Can you work these out from the model? Positions are in its coordinate system, mm. A direction names the side the tool comes from. Coordinates: 2 decimals unless noted, no trailing zeros. Order: outer loops, then holes, each group sorted by start corner. A loop starts at its lowest first (then second) coordinate and runs counter-clockwise, first axis right, second up. Notation, with made-up numbers: (6.25, 80.5) -> (34.25, 80.5) arc R15 cw to (34.25, 104.5) -> close; hole circle Ø10 at (65, -35.5). An arc over 180 degrees is marked (long way). Return JSON: item names as keys, results as strings. Group by question number.
1) Thinking about a two-plate mould opening in Y: for faces 5 (the flat face through (-8.65, 0, 6)), 6 (the cylindrical face through (-9.04, -9, 2.03)), 7 (the flat face through (0, 9.9, 2)), 8 (the flat face through (-9.9, 0, 2)), which applies, +Y half, -Y half, draft (parallel to the pull), parting line (faces both ways), or undercut?
2) If we section it at B-B, the plane y = -4.25: Please give me the cut outline in (x, z), then the cut area to 3 significant figures.
3) If we section it at A-A, the plane x = 0.75: Please give me the cut outline in (y, z).
4) For faces 1 (the flat face through (-8.4, 7, 1)), 2 (the flat face through (4.1, 0, 3)), 3 (the flat face through (8.35, 7, 6)), 4 (the flat face through (0, 9.55, 6)), which set-ups out of +Z, -Z, +X, -X, +Y, -Y let a thin tool reach every point of the face, with its end or its side?
5) If we section it at D-D, the plane z = 3.5: Please give me the cut outline in (x, y).
6) If I drill on probe 1 along Y at (x, z) = (-5.5, 2.5); probe 2 along X at (y, z) = (1, 0.5); probe 3 along Y at (x, z) = (-0.75, 5.5), over which ranges is the centre line in solid material (lowest first)? Write a range as from..to.
7) If we section it at C-C, the plane z = 5.5: Please give me the cut outline in (x, y).
8) For pin 1 (1 mm diameter, centred on y = 7, z = 1, fed in from +X); pin 2 (4 mm diameter, centred on y = 3, z = 1, fed in from -X); pin 3 (1.5 mm diameter, centred on x = -4.5, y = -4, fed in from +Z); pin 4 (0.6 mm diameter, centred on x = -4, z = 6, fed in from +Y), each with a flat end and sliding along its axis, tell me the tip position at first contact or that it passes through.
Autodesk Fusion 360 part; units mm, degrees
sketch "Sketch1" plane through (0, 0, 0) normal (0, 0, 1) x (1, 0, 0)
  line L0 (9.9, 9.9) -> (-9.9, 9.9)
  line L1 (-9.9, 9.9) -> (-9.9, -9.9)
  line L2 (-9.9, -9.9) -> (9.9, -9.9)
  line L3 (9.9, -9.9) -> (9.9, 9.9)
  line L4 (9.9, 9.9) -> (-9.9, -9.9) construction
  line L5 (-9.9, 9.9) -> (9.9, -9.9) construction
  line L6 (11, -11) -> (-11, -11)
  line L7 (-11, -11) -> (-11, 11)
  line L8 (-11, 11) -> (11, 11)
  line L9 (11, 11) -> (11, -11)
  line L10 (11, -11) -> (-11, 11) construction
  line L11 (-11, -11) -> (11, 11) construction
  line L12 (8.9, -8.9) -> (-8.9, -8.9)
  line L13 (-8.9, -8.9) -> (-8.9, 8.9)
  line L14 (-8.9, 8.9) -> (8.9, 8.9)
  line L15 (8.9, 8.9) -> (8.9, -8.9)
  line L16 (8.9, -8.9) -> (-8.9, 8.9) construction
  line L17 (-8.9, -8.9) -> (8.9, 8.9) construction
  line L18 (8.4, -6) -> (-8.4, -6)
  line L19 (-8.4, -6) -> (-8.4, 6)
  line L20 (-8.4, 6) -> (8.4, 6)
  line L21 (8.4, 6) -> (8.4, -6)
  line L22 (8.4, -6) -> (-8.4, 6) construction
  line L23 (-8.4, -6) -> (8.4, 6) construction
  line L24 (8.0957, 8.0957) -> (-8.0957, 8.0957)
  line L25 (-8.0957, 8.0957) -> (-8.0957, -8.0957)
  line L26 (-8.0957, -8.0957) -> (8.0957, -8.0957)
  line L27 (8.0957, -8.0957) -> (8.0957, 8.0957)
  line L28 (8.0957, 8.0957) -> (-8.0957, -8.0957) construction
  line L29 (-8.0957, 8.0957) -> (8.0957, -8.0957) construction
  line L30 (8.9, -0.5) -> (-8.9, -0.5)
  line L31 (-8.9, -0.5) -> (-8.9, 0.5)
  line L32 (-8.9, 0.5) -> (8.9, 0.5)
  line L33 (8.9, 0.5) -> (8.9, -0.5)
  line L34 (8.9, -0.5) -> (-8.9, 0.5) construction
  line L35 (-8.9, -0.5) -> (8.9, 0.5) construction
  dimension "d1" = 19.8
  dimension "d2" = 19.8
  dimension "d3" = 22
  dimension "d4" = 22
  dimension "d5" = 17.8
  dimension "d6" = 17.8
  dimension "d7" = 16.8
  dimension "d8" = 12
  dimension "d53" = 1
extrude "Extrude1" add sketch "Sketch1" along normal blind 1 contours L12 L13 L15 L18 L19 L21 L25 L26 L27 L30 | L15 L21 L30 L32 L33 | L13 L19 L30 L31 L32 | L13 L14 L15 L19 L20 L21 L24 L25 L27 L32 | L18 L25 L26 L27 | L20 L24 L25 L27
extrude "Extrude2" add sketch "Sketch1" along normal blind 4 contours L0 L1 L2 L3
extrude "Extrude3" add sketch "Sketch1" along normal blind 5 contours L6 L7 L8 L9
extrude "Extrude4" cut sketch "Sketch1" along normal blind 4 contours L6 L7 L8 L9
extrude "Extrude5" add 1 faces at (-9.5667, -2.9667, 4) along direction (0, 0, 1) blind 1
fillet "Fillet1" radius 3 1 edges at (9.9, -9.9, 2)
fillet "Fillet2" radius 3 1 edges at (-9.9, -9.9, 2)
fillet "Fillet3" radius 3 2 edges at (-9.9, 9.9, 2) (9.9, 9.9, 2)
fillet "Fillet4" radius 1 4 edges at (-11, -11, 4.5) (-11, 11, 4.5) (11, -11, 4.5) (11, 11, 4.5)
extrude "Extrude6" add 1 faces at (-2.8, -7.9333, 1) along direction (0, 0, 1) blind 5
extrude "Extrude7" cut sketch "Sketch1" along normal blind 3 contours L18 L25 L26 L27 | L20 L24 L25 L27
extrude "Extrude8" cut 1 faces at (-8.0957, 7.3972, 1) along direction (-1, 0, 0) blind 0.304
extrude "Extrude9" cut 1 faces at (8.0957, 6.6986, 1) along direction (1, 0, 0) blind 0.304
extrude "Extrude10" cut 1 faces at (8.0957, -7.3972, 1) along direction (1, 0, 0) blind 0.304
extrude "Extrude11" cut 1 faces at (-8.0957, -6.6986, 1) along direction (-1, 0, 0) blind 0.304
sketch "Sketch2" plane through (8.4, 0, 0) normal (-1, 0, 0) x (0, -1, 0)
  line L0 (-6, 0) -> (6, 0)
  line L1 (6, 0) -> (6, 6)
  line L2 (6, 6) -> (-6, 6)
  line L3 (-6, 6) -> (-6, 0)
  line L4 (-6, 6) -> (6, 6)
  line L5 (6, 6) -> (6, 4.0166)
  line L6 (6, 4.0166) -> (-6, 4.0166)
  line L7 (-6, 4.0166) -> (-6, 6)
extrude "Extrude12" add sketch "Sketch2" along normal blind 1 contours L1 L2 L3 L4 L5 L6 L7
sketch "Sketch3" plane through (-8.4, 0, 0) normal (1, 0, 0) x (0, 1, 0)
  line L0 (-6, 0) -> (6, 0)
  line L1 (6, 0) -> (6, 6)
  line L2 (6, 6) -> (-6, 6)
  line L3 (-6, 6) -> (-6, 0)
  line L4 (-6, 6) -> (6, 6)
  line L5 (6, 6) -> (6, 3.9624)
  line L6 (6, 3.9624) -> (-6, 3.9624)
  line L7 (-6, 3.9624) -> (-6, 6)
extrude "Extrude13" add sketch "Sketch3" along normal blind 1 contours L1 L2 L3 L4 L5 L6 L7
extrude "Extrude14" cut 1 faces at (-2.4667, 7.9333, 6) along direction (0, 0, -1) blind 2
extrude "Extrude15" add 1 faces at (-2.4667, 7.9333, 4) along direction (0, 0, 1) blind 1
sketch "TOP BUTTON GUIDE" plane through (0, 0, 5) normal (0, 0, 1) x (-1, 0, 0)
  line L0 (-8.4, 6) -> (7.4, 6)
  line L1 (7.4, 6) -> (7.4, -6)
  line L2 (7.4, -6) -> (-8.4, -6)
  line L3 (-8.4, -6) -> (-8.4, 6)
  arc A0 (-11, -10) -> (-10, -11) centre (-10, -10) ccw
  line L4 (-10, -11) -> (10, -11)
  arc A1 (10, -11) -> (11, -10) centre (10, -10) ccw
  line L5 (11, -10) -> (11, 10)
  arc A2 (11, 10) -> (10, 11) centre (10, 10) ccw
  line L6 (10, 11) -> (-10, 11)
  arc A3 (-10, 11) -> (-11, 10) centre (-10, 10) ccw
  line L7 (-11, 10) -> (-11, -10)
  line L8 (-8.35, 8.25) -> (8.35, 8.25)
  line L9 (8.35, 8.25) -> (8.35, -8.25)
  line L10 (8.35, -8.25) -> (-8.35, -8.25)
  line L11 (-8.35, -8.25) -> (-8.35, 8.25)
  line L12 (-8.35, 8.25) -> (8.35, -8.25) construction
  line L13 (8.35, 8.25) -> (-8.35, -8.25) construction
  line L14 (-9.15, 9.05) -> (9.15, 9.05)
  line L15 (9.15, 9.05) -> (9.15, -9.05)
  line L16 (9.15, -9.05) -> (-9.15, -9.05)
  line L17 (-9.15, -9.05) -> (-9.15, 9.05)
  line L18 (-9.15, 9.05) -> (9.15, -9.05) construction
  line L19 (9.15, 9.05) -> (-9.15, -9.05) construction
  dimension "d47" = 16.7
  dimension "d48" = 16.5
  dimension "d49" = 18.3
  dimension "d50" = 18.1
extrude "Extrude16" add sketch "TOP BUTTON GUIDE" along normal blind 2 contours L14 L15 L16 L17
extrude "Extrude17" add sketch "Sketch1" along normal blind 5 contours L21 L27 L30 L32 | L19 L25 L30 L32 | L25 L27 L30 L32
sketch "Sketch5" plane through (0, 0, 5) normal (0, 0, 1) x (-1, 0, 0)
  line L0 (7.4, -0.5) -> (7.4, -6)
  line L1 (7.4, -6) -> (-8.35, -6)
  line L2 (-8.35, -6) -> (-8.35, -8.25)
  line L3 (-8.35, -8.25) -> (8.35, -8.25)
  line L4 (8.35, -8.25) -> (8.35, 8.25)
  line L5 (8.35, 8.25) -> (-8.35, 8.25)
  line L6 (-8.35, 8.25) -> (-8.35, 6)
  line L7 (-8.35, 6) -> (7.4, 6)
  line L8 (7.4, 6) -> (7.4, 0.5)
  line L9 (7.4, 0.5) -> (-8.4, 0.5)
  line L10 (-8.4, 0.5) -> (-8.4, -0.5)
  line L11 (-8.4, -0.5) -> (7.4, -0.5)
  line L12 (-3.5, 1.3147) -> (3.5, 1.3147)
  line L13 (3.5, 1.3147) -> (3.5, -1.3147)
  line L14 (3.5, -1.3147) -> (-3.5, -1.3147)
  line L15 (-3.5, -1.3147) -> (-3.5, 1.3147)
  line L16 (-3.5, 1.3147) -> (3.5, -1.3147) construction
  line L17 (3.5, 1.3147) -> (-3.5, -1.3147) construction
  dimension "d56" = 7
extrude "Extrude18" cut sketch "Sketch5" against normal blind 6 contours L9 L11 L13 L15
extrude "Extrude19" cut 1 faces at (-2.7833, 8.25, 5.6667) along direction (0, 1, 0) blind 0.5
extrude "Extrude20" add 1 faces at (-3.05, 9.05, 5.6667) along direction (0, 1, 0) blind 0.5
extrude "Extrude21" cut 1 faces at (-8.35, 3.0833, 6.3333) along direction (-1, 0, 0) blind 0.3
extrude "Extrude22" add 1 faces at (-9.15, 3.35, 5.6667) along direction (-1, 0, 0) blind 0.3
sketch "Sketch6" plane through (0, 0, 5) normal (0, 0, 1) x (-1, 0, 0)
  line L0 (3.5, 0.5) -> (3.5, -0.5)
  line L1 (3.5, -0.5) -> (7.4, -0.5)
  line L2 (7.4, -0.5) -> (7.4, -6)
  line L3 (7.4, -6) -> (-8.35, -6)
  line L4 (-8.35, -6) -> (-8.35, -8.75)
  line L5 (-8.35, -8.75) -> (8.65, -8.75)
  line L6 (8.65, -8.75) -> (8.65, 8.25)
  line L7 (8.65, 8.25) -> (-8.35, 8.25)
  line L8 (-8.35, 8.25) -> (-8.35, 6)
  line L9 (-8.35, 6) -> (7.4, 6)
  line L10 (7.4, 6) -> (7.4, 0.5)
  line L11 (7.4, 0.5) -> (3.5, 0.5)
  circle A0 centre (6.4473, -6.6661) radius 0.4424
extrude "Extrude23" cut sketch "Sketch6" against normal blind 2 contours A0
extrude "Extrude24" cut 1 faces at (-3.5, -0.1667, 3.3333) along direction (-1, 0, 0) blind 0.6
extrude "Extrude25" cut 1 faces at (3.5, 0.1667, 3.3333) along direction (1, 0, 0) blind 0.6
Result sheet:
{
 "1": {"face 5": "undercut", "face 6": "-Y half", "face 7": "+Y half", "face 8": "draft"},
 "2": {"outline": "(-11, 4) -> (-9.9, 4) -> (-9.9, 0) -> (-8.4, 0) -> (-8.4, 3.96) -> (-7.4, 3.96) -> (-7.4, 5) -> (-8.65, 5) -> (-8.65, 7) -> (-9.45, 7) -> (-9.45, 5) -> (-11, 5) -> close; (8.4, 0) -> (9.9, 0) -> (9.9, 4) -> (11, 4) -> (11, 5) -> (9.15, 5) -> (9.15, 7) -> (8.4, 7) -> close", "area": "21.3 mm2"},
 "3": {"outline": "(-11, 4) -> (-9.9, 4) -> (-9.9, 0) -> (-8.1, 0) -> (-8.1, 3) -> (-6, 3) -> (-6, 5) -> (-8.25, 5) -> (-8.25, 7) -> (-9.05, 7) -> (-9.05, 5) -> (-11, 5) -> close; (6, 3) -> (8.1, 3) -> (8.1, 0) -> (9.9, 0) -> (9.9, 4) -> (11, 4) -> (11, 5) -> (9.55, 5) -> (9.55, 7) -> (8.75, 7) -> (8.75, 5) -> (6, 5) -> close"},
 "4": {"face 1": "-Z", "face 2": "+Z, -Z", "face 3": "+Z", "face 4": "+Z, +X, -X, +Y"},
 "5": {"outline": "(-9.9, -6.9) arc R3 ccw to (-6.9, -9.9) -> (6.9, -9.9) arc R3 ccw to (9.9, -6.9) -> (9.9, 6.9) arc R3 ccw to (6.9, 9.9) -> (-6.9, 9.9) arc R3 ccw to (-9.9, 6.9) -> close; hole (-8.4, -6) -> (8.4, -6) -> (8.4, -0.5) -> (4.1, -0.5) -> (4.1, 0.5) -> (8.4, 0.5) -> (8.4, 6) -> (-8.4, 6) -> (-8.4, 0.5) -> (-4.1, 0.5) -> (-4.1, -0.5) -> (-8.4, -0.5) -> close; hole circle Ø0.88 at (-6.45, 6.67)"},
 "6": {"probe 1": "y = -9.9..-8.1, -0.5..0.5, 8.1..9.9", "probe 2": "x = -9.9..-8.4, 8.4..9.9", "probe 3": "y = -9.05..-8.25, 8.75..9.55"},
 "7": {"outline": "(-9.45, -9.05) -> (9.15, -9.05) -> (9.15, 9.55) -> (-9.45, 9.55) -> close; hole (-8.65, -8.25) -> (8.35, -8.25) -> (8.35, -6) -> (8.4, -6) -> (8.4, 6) -> (8.35, 6) -> (8.35, 8.75) -> (-8.65, 8.75) -> close"},
 "8": {"pin 1": "stops at x = 9.9", "pin 2": "stops at x = -9.9", "pin 3": "passes through", "pin 4": "stops at y = 9.55"}
}
